The figure shows three views and two pictorial views of one solid part (mm, origin at its lowest corner). Answer the questions. Round coordinates to 2 decimals unless told otherwise and drop trailing zeros. Order: outer loops, then holes, each group sorted by start corner. A loop starts at its lowest first (then second) coordinate and runs counter-clockwise, first axis right, second up. Notation, with made-up numbers: (72, 23.25) -> (96, 23.25) arc R22 cw to (96, 36.25) -> close; hole circle Ø3 at (48, 1.5). An arc over 180 degrees is marked (long way). Return JSON: item names as keys, results as strings. Group by question number.
(1) Consider line 1 (Z direction, x = 27.5, y = 3); line 2 (Z direction, x = 29.5, y = 5.35) (1 decimal); line 3 (X direction, y = 0.3, z = 10.5) (1 decimal). Determine where each line is inside the solid, lowest interval first. Write a range as [from, to].
(2) Determine the mould class of the marked faces 1, 2 and 3 for opening direction X: +X half, -X half, draft (parallel to the pull), parting line (faces both ways), or undercut.
(3) The part is cut by section B-B (x = 27.5). Determine the outline of the cut face in (y, z), plus the area to 3 significant figures.
(4) The part is cut by section C-C (z = 47.5). Determine the outline of the cut face in (x, y).
(5) The part is cut by section D-D (x = 7.5). Determine the outline of the cut face in (y, z).
(6) The part is cut by section A-A (z = 27.5). Determine the outline of the cut face in (x, y).
(7) Each of these flat-tipped pins is pushed along its axis until it touches: pin 1 (7.5 mm diameter, centred on x = 13.36, z = 41.64, fed in from -Y); pin 2 (3 mm diameter, centred on x = 25, y = 1.5, fed in from -Z); pin 3 (5.5 mm diameter, centred on x = 47.5, z = 27.5, fed in from -Y); pin 4 (2 mm diameter, centred on x = 30, y = 4.5, fed in from +Z). Where does it stop, or does it pass through?
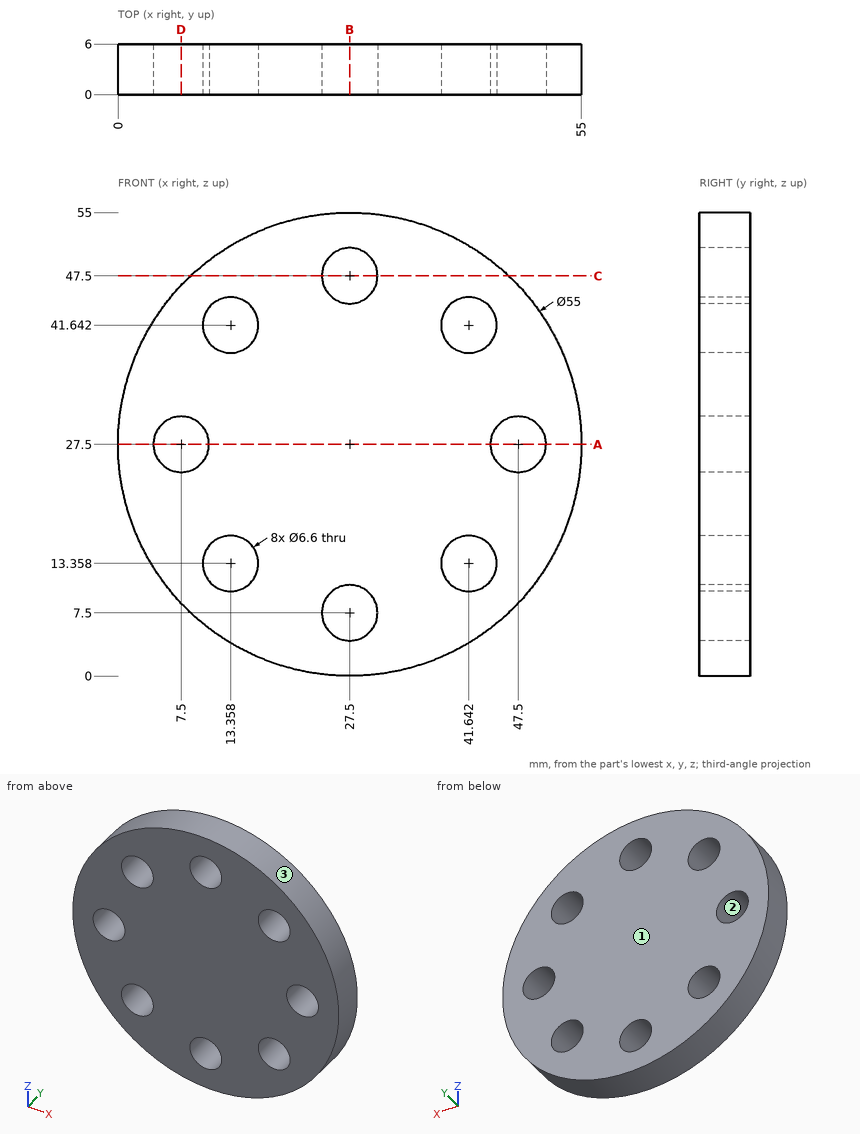
Answer below:
{
 "1": {"line 1": "z = [0, 4.2], [10.8, 44.2], [50.8, 55]", "line 2": "z = [0.1, 4.9], [10.1, 44.9], [50.1, 54.9]", "line 3": "x = [5.9, 11.7], [15, 26.1], [28.9, 40], [43.3, 49.1]"},
 "2": {"face 1": "draft", "face 2": "undercut", "face 3": "parting line"},
 "3": {"outline": "(0, 0) -> (6, 0) -> (6, 4.2) -> (0, 4.2) -> close; (0, 10.8) -> (6, 10.8) -> (6, 44.2) -> (0, 44.2) -> close; (0, 50.8) -> (6, 50.8) -> (6, 55) -> (0, 55) -> close", "area": "251 mm²"},
 "4": {"outline": "(8.63, 0) -> (24.2, 0) -> (24.2, 6) -> (8.63, 6) -> close; (30.8, 0) -> (46.37, 0) -> (46.37, 6) -> (30.8, 6) -> close"},
 "5": {"outline": "(0, 8.63) -> (6, 8.63) -> (6, 24.2) -> (0, 24.2) -> close; (0, 30.8) -> (6, 30.8) -> (6, 46.37) -> (0, 46.37) -> close"},
 "6": {"outline": "(0, 0) -> (4.2, 0) -> (4.2, 6) -> (0, 6) -> close; (10.8, 0) -> (44.2, 0) -> (44.2, 6) -> (10.8, 6) -> close; (50.8, 0) -> (55, 0) -> (55, 6) -> (50.8, 6) -> close"},
 "7": {"pin 1": "stops at y = 0", "pin 2": "stops at z = 0.02", "pin 3": "passes through", "pin 4": "stops at z = 54.96"}
}
